Geometry: final body of the model. Coordinates: model frame, mm. Face numbers are marked on the shaded views. A direction names the side the tool comes from. Give positions to 0.01 mm unless a question says otherwise; leave off trailing zeros. Loops run counter-clockwise (first coordinate to the right, second up) from the corner with the lowest first, then second, coordinate; pieces in that order, holes last. Notation, with made-up numbers: (-15.5, 21.25) - (36.5, 21.25) arc R21 ccw to (36.5, 53.25) - close; hole circle Ø5 at (32, -14). An arc over 180 degrees is marked (long way). Use one line per item in the form item = value.
Autodesk Inventor part; units mm, degrees
ref_plane "Work Plane1" through (0, 0, -15) normal (0, 0, 1) x (1, 0, 0)
ref_plane "YZ Plane" through (0, 0, 0) normal (1, 0, 0) x (0, 1, 0)
ref_plane "XZ Plane" through (0, 0, 0) normal (0, 1, 0) x (-1, 0, 0)
sketch "Sketch1" plane through (0, 0, 0) normal (0, 0, 1) x (1, 0, 0)
  line L0 (0, 0) -> (25, 0)
  line L1 (25, 0) -> (25, 40)
  line L2 (25, 40) -> (0, 40)
  line L3 (0, 40) -> (0, 0)
  dimension "d1" = 25
  dimension "d2" = 40
  dimension "d3" = 25
extrude "Extrusion1" add sketch "Sketch1" against normal blind 30
sketch "Sketch2" plane through (25, 0, 0) normal (1, 0, 0) x (0, 0, -1)
  line L0 (0, 0) -> (30, 0)
  circle A0 centre (15, 6.56) radius 2.46
extrude "Extrusion2" cut sketch "Sketch2" against normal blind 30
sketch "Sketch3" plane through (0, 0, 0) normal (-1, 0, 0) x (0, 0, 1)
  line L0 (0, 0) -> (-30, 0)
  line L1 (-25.05, 0) -> (-4.95, 0)
  line L2 (-4.95, 0) -> (-4.95, 33.12)
  line L3 (-4.95, 33.12) -> (-25.05, 33.12)
  line L4 (-25.05, 33.12) -> (-25.05, 0)
  dimension "d11" = 20.1
extrude "Extrusion3" cut sketch "Sketch3" against normal blind 20
sketch "Sketch4" plane through (0, 0, 0) normal (0, -1, 0) x (1, 0, 0)
  line L0 (20, -4.95) -> (20, -25.05)
  line L1 (20, -15) -> (25, -15)
  line L2 (25, 0) -> (25, -30)
  line L3 (20, -8.025) -> (25, -8.025)
  line L4 (25, -8.025) -> (25, -21.975)
  line L5 (25, -21.975) -> (20, -21.975)
  line L6 (20, -21.975) -> (20, -8.025)
  line L7 (20, -8.025) -> (25, -21.975) construction
  line L8 (25, -8.025) -> (20, -21.975) construction
  line L9 (25, -12.54) -> (25, -17.46)
  point P0 (0, 0)
  point P1 (22.5, -15)
  dimension "d14" = 13.95
extrude "Extrusion4" add sketch "Sketch4" along normal blind 15
sketch "Sketch5" plane through (20, 0, 0) normal (-1, 0, 0) x (0, 0, 1)
  circle A0 centre (-15, 6.56) radius 2.46
  circle A1 centre (-15, 6.56) radius 4.7025
  circle A2 centre (-15, 6.56) radius 2.46
  circle A3 centre (-15, 6.56) radius 2.46
  point P0 (0, 0)
  dimension "d17" = 9.405
extrude "Extrusion5" cut sketch "Sketch5" against normal blind 2.1
sketch "Sketch6" plane through (25, 0, 0) normal (1, 0, 0) x (0, 0, -1)
  circle A0 centre (15, 6.56) radius 4.7025
  line L0 (15, 6.56) -> (15, 23.56)
  circle A1 centre (15, 23.56) radius 2.46
  point P0 (0, 0)
  dimension "d20" = 17
  dimension "d21" = 4.92
extrude "Extrusion6" cut sketch "Sketch6" against normal blind 10 contours A1
sketch "Sketch7" plane through (20, 0, 0) normal (-1, 0, 0) x (0, 0, 1)
  circle A0 centre (-15, 23.56) radius 2.46
  circle A1 centre (-15, 23.56) radius 4.7025
  point P0 (0, 0)
  dimension "d24" = 9.405
extrude "Extrusion7" cut sketch "Sketch7" against normal blind 2.1
sketch "Sketch9" plane through (25, 0, 0) normal (1, 0, 0) x (0, 0, -1)
  circle A0 centre (15, 6.56) radius 2.46
  circle A1 centre (15, 6.56) radius 2.46
  circle A2 centre (15, 23.56) radius 2.46
  circle A3 centre (15, 23.56) radius 2.46
  line L0 (30, 40) -> (30, 0)
  line L1 (30, 0) -> (30, 40)
  line L2 (30, 40) -> (0, 40)
  line L3 (0, 40) -> (0, 0)
  line L4 (0, 0) -> (8.025, 0)
  line L5 (21.975, 0) -> (21.975, -15)
  line L6 (21.975, -15) -> (8.025, -15)
  line L7 (8.025, -15) -> (8.025, 0)
  line L8 (0, 0) -> (8.025, 0)
  line L9 (21.975, 0) -> (30, 0)
extrude "Extrusion8" add sketch "Sketch9" along normal blind 5
sketch "Sketch10" plane through (0, 40, 0) normal (0, 1, 0) x (1, 0, 0)
  line L0 (0, 30) -> (30, 30)
  line L1 (30, 0) -> (0, 0)
  line L2 (0, 30) -> (30, 30)
  line L3 (30, 30) -> (30, 0)
  line L4 (30, 0) -> (0, 0)
  line L5 (0, 0) -> (0, 30)
extrude "Extrusion9" add sketch "Sketch10" along normal blind 30
sketch "Sketch12" plane through (30, 0, 0) normal (1, 0, 0) x (0, 0, -1)
  circle A0 centre (15, 6.56) radius 2.46
  line L0 (15, 6.56) -> (15, 15.06)
  circle A1 centre (15, 15.06) radius 2.525
  point P0 (0, 0)
  dimension "d31" = 8.5
  dimension "d33" = 5.05
extrude "Extrusion10" cut sketch "Sketch12" against normal blind 30 contours A1
sketch "Sketch14" plane through (0, 0, 0) normal (0, 0, 1) x (1, 0, 0)
  line L0 (30, 70) -> (0, 70)
  line L1 (0, 70) -> (0, 85)
  line L2 (30, 0) -> (30, 70)
  line L3 (30, 113) -> (30, 70)
  line L4 (30, 105) -> (30, 100)
  line L5 (-12, 128) -> (15, 128)
  line L6 (-8, 126) -> (-12, 128)
  line L7 (-8, 126) -> (-4, 114)
  line L8 (-8, 102) -> (-12, 100)
  line L9 (-8, 102) -> (-4, 114)
  line L10 (30, 113) -> (15, 128)
  line L11 (0, 100) -> (-12, 100)
  line L12 (0, 100) -> (0, 85)
  point P0 (0, 0)
  dimension "d69" = 28
  dimension "d74" = 12
extrude "Extrusion12" add sketch "Sketch14" against normal blind 30
sketch "Sketch15" plane through (0, 0, -25.05) normal (-1, 0, 0) x (0, 0, 1)
  line L0 (0, 33.12) -> (20.1, 33.12)
  line L1 (20.1, 33.12) -> (20.1, 0)
  line L2 (0, 33.12) -> (20.1, 33.12)
  line L3 (20.1, 33.12) -> (20.1, 31.1)
  line L4 (20.1, 31.1) -> (0, 31.1)
  line L5 (0, 31.1) -> (0, 33.12)
  point P0 (25.05, 0)
  dimension "d57" = 2.02
extrude "Extrusion13" add sketch "Sketch15" against normal blind 20
sketch "Sketch21" plane through (0, 0, 0) normal (0, 0, 1) x (1, 0, 0)
  line L0 (0, 100) -> (-12, 100)
  line L1 (0, 100) -> (-12, 100)
  line L2 (-12, 100) -> (-8, 102)
  line L3 (-12, 100) -> (-8, 102)
  line L4 (-8, 102) -> (-4, 114)
  line L5 (-8, 102) -> (-4, 114)
  line L6 (-4, 114) -> (-8, 126)
  line L7 (-4, 114) -> (-8, 126)
  line L8 (-8, 126) -> (-12, 128)
  line L9 (-8, 126) -> (-12, 128)
  line L10 (-12, 128) -> (15, 128)
  line L11 (-12, 128) -> (15, 128)
  line L12 (15, 128) -> (30, 113)
  line L13 (15, 128) -> (30, 113)
  line L14 (30, 113) -> (30, 93)
  line L15 (30, 0) -> (30, 113)
  line L16 (30, 93) -> (0, 93)
  line L17 (0, 93) -> (0, 100)
  point P0 (0, 0)
  dimension "d75" = 20
  dimension "d76" = 30
extrude "Extrusion14" add sketch "Sketch21" along normal blind 15
ref_plane "Work Plane1" through (0, 0, -15) normal (0, 0, 1) x (1, 0, 0)
mirror "Mirror1" about plane through (0, 0, -15) normal (0, 0, 1) of "Extrusion14"
properties part number "rec_b_24mm_x_60mm"
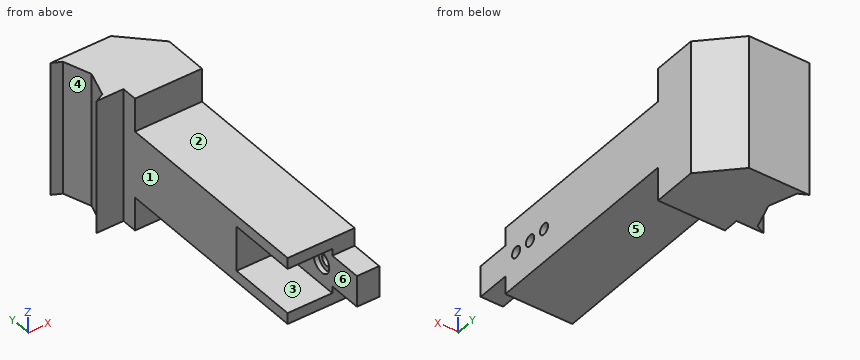
(1) Material intervals for L1, parallel to Z at x = 16, y = 9; L2, parallel to Z at x = 27.5, y = 23.56; L3, parallel to Y at x = 21, z = -15 (1 decimal), sorted ascending. Write a range as from..to.
Solution:
L1 = -30..-25.05, -4.95..0
L2 = -30..-17.46, -12.54..0
L3 = -15..1.9, 11.3..12.5, 17.6..18.9, 28.3..122
(2) Cut plane D-D (z = 10). Return the cut outline in (x, y).
Solution:
outline = (-12, 100) - (0, 100) - (0, 93) - (30, 93) - (30, 113) - (15, 128) - (-12, 128) - (-8, 126) - (-4, 114) - (-8, 102) - close
(3) Cut plane A-A (y = 15.06). Return the cut outline in (x, z) (3 decimals), plus the area to 4 significant figures.
Solution:
outline = (0, -30) - (30, -30) - (30, -17.525) - (20, -17.525) - (20, -25.05) - (0, -25.05) - close; (0, -4.95) - (20, -4.95) - (20, -12.475) - (30, -12.475) - (30, 0) - (0, 0) - close
area = 447.5 mm2
(4) Pull-direction query (Z, two-part tool) for the marked faces 1, 2 and 3; classes: released by +Z, released by -Z, zero draft, split by the parting line, or undercut.
Solution:
face_1 = zero draft
face_2 = released by +Z
face_3 = undercut
(5) Access query for the marked faces 4, 5 and 6. Directions: +Z, -Z, +X, -X, +Y, -Y. A direction counts if a zero-diameter tool reaches every point of the face in a straight line with its end or side. Return the directions, or none.
Solution:
face_4 = +Z, -Z, -X
face_5 = -Z, +X, -X, -Y
face_6 = -X, -Y
(6) Cut plane B-B (z = -15). Give the number of separate pieces and of enclosed holes in the cut face, plus the area to 3 significant figures.
Solution:
separate_pieces = 4
enclosed_holes = 0
area = 3,270 mm2
(7) Cut plane C-C (x = 13). Return the cut outline in (y, z), plus the area to 3 significant figures.
Solution:
outline = (0, -30) - (93, -30) - (93, -45) - (128, -45) - (128, 15) - (93, 15) - (93, 0) - (0, 0) - (0, -4.95) - (31.1, -4.95) - (31.1, -25.05) - (0, -25.05) - close
area = 4,260 mm2
(8) Pin query (flat end, axial travel): P1, Ø10, axis at x = 25, y = 21, coming from the +Z side; P2, Ø4.5, axis at x = 8, z = 4.5, coming from the -Y side; P3, Ø2, axis at y = 83.5, z = -7, coming from the -X side. Return the tip coordinate at first contact, or that it passes through.
Solution:
P1 = 0
P2 = 93
P3 = 0
